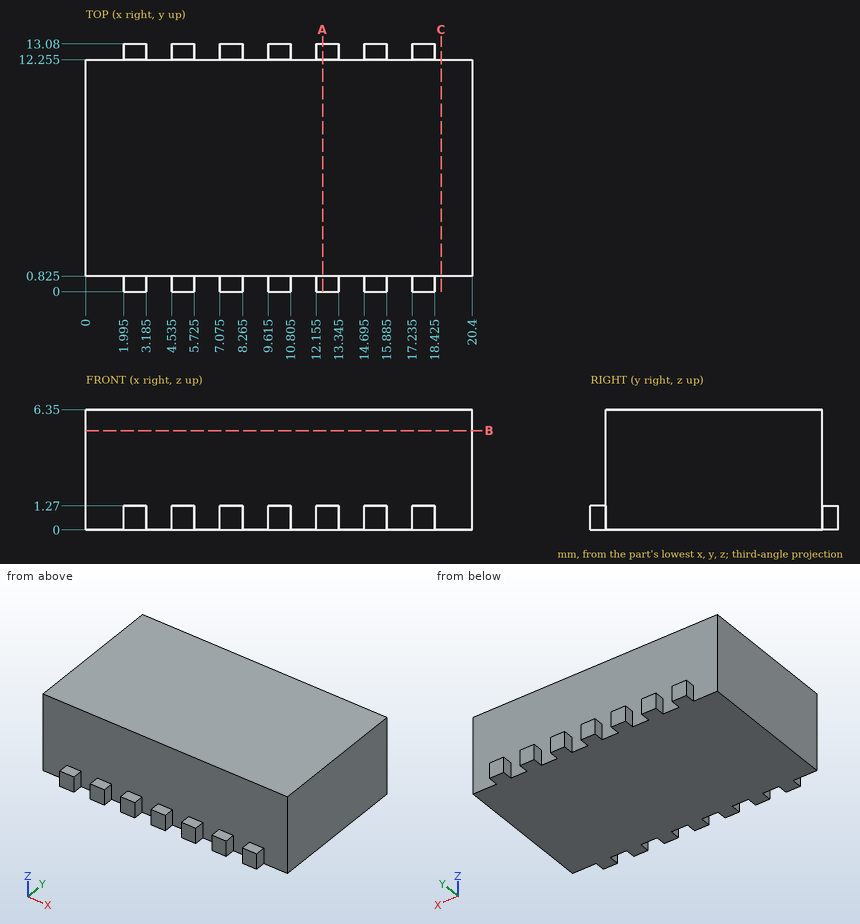
For this review, use the dimensioned drawing (mm, ordinates from the lowest corner) and the shaded views. Round coordinates to 2 decimals unless told otherwise and drop trailing zeros. Write each loop counter-clockwise with the first axis right and the second up, starting at its lowest first coordinate (ties: lowest second). Pieces come first, ordered by that corner, then holes. Notation, with made-up numbers: M 38.25,-14 L 86.25,-14 A8 ccw 86.25,-6 Z; hole C -32.75,61 d5. An arc over 180 degrees is marked long. Use CSV: the item, a comma, the result in double quotes. Start each with the question number.
(1) We need section C-C, the plane x = 18.75. State the section outline as (y, z) points (3 decimals), then the cut area to 3 significant figures.
(2) We need section B-B, the plane z = 5.25. State the section outline as (x, y) points (3 decimals).
(3) We need section A-A, the plane x = 12.5. State the section outline as (y, z) points (3 decimals).
(4) For line 1 along Y through (x, z) = (13.5, 3.5) (3 decimals), list the stretches that pass through material, from the lowest coordinate up.
(5) Clearance check with flat-ended pins moving along their axes: P1, Ø3, axis at y = 8.5, z = 3.5, coming from the -X side; P2, Ø0.7, axis at y = 13, z = 0.5, coming from the +X side (3 decimals); P3, Ø1, axis at x = 4, z = 4.5, coming from the +Y side (3 decimals); P4, Ø0.9, axis at y = 13, z = 0.5, coming from the -X side (3 decimals). State where each tip first meets the part, or that it passes through.
Findings:
1,outline,"M 0.825,0 L 12.255,0 L 12.255,6.35 L 0.825,6.35 Z"
1,area,"72.6 mm^2"
2,outline,"M 0,0.825 L 20.4,0.825 L 20.4,12.255 L 0,12.255 Z"
3,outline,"M 0,0 L 13.08,0 L 13.08,1.27 L 12.255,1.27 L 12.255,6.35 L 0.825,6.35 L 0.825,1.27 L 0,1.27 Z"
4,line 1,"0.825 to 12.255"
5,P1,"x = 0"
5,P2,"x = 18.425"
5,P3,"y = 12.255"
5,P4,"x = 1.995"
